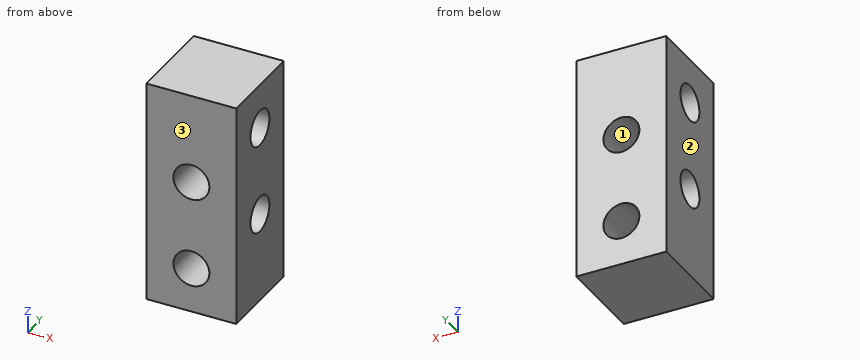
from build123d import *

# Parameters (mm, degrees)
SKETCH_1_W          = 10
SKETCH_1_H          = 10
EXTRUDE_1_DEPTH     = 12.5
SKETCH_2_R          = 2
CUT_EXTRUDE_1_DEPTH = 25
SKETCH_3_R          = 2
CUT_EXTRUDE_2_DEPTH = 25


with BuildPart() as part:
    # 草图1 → 凸台-拉伸1 (new body, symmetric)
    with BuildSketch(Plane.XY):
        Rectangle(SKETCH_1_W, SKETCH_1_H)
    extrude(amount=EXTRUDE_1_DEPTH, both=True)

    # 草图2 → 切除-拉伸1 (cut)
    with BuildSketch(Plane(origin=(5, 0, 0), x_dir=(0, 0, -1), z_dir=(1, 0, 0))):
        with Locations((-7.5, 0)):
            Circle(SKETCH_2_R)
        with Locations((2.5, 0)):
            Circle(SKETCH_2_R)
    extrude(amount=-CUT_EXTRUDE_1_DEPTH, mode=Mode.SUBTRACT)

    # 草图3 → 切除-拉伸2 (cut)
    with BuildSketch(Plane(origin=(0, 5, 0), x_dir=(1, 0, 0), z_dir=(0, 1, 0))):
        with Locations((0, 7.5)):
            Circle(SKETCH_3_R)
        with Locations((0, -2.5)):
            Circle(SKETCH_3_R)
    extrude(amount=-CUT_EXTRUDE_2_DEPTH, mode=Mode.SUBTRACT)


solid = part.part
Geometry: final body of the model. Coordinates: model frame, mm. Face numbers are marked on the shaded views. Give positions to 0.01 mm unless a question says otherwise; leave off trailing zeros. Write each loop counter-clockwise with the first axis right and the second up, starting at its lowest first coordinate (ties: lowest second). Pieces come first, ordered by that corner, then holes.
(1) Mould query, pull axis X, two halves, no side actions, for the marked faces 1, 2 and 3. Classes: released by +X, released by -X, zero draft, split by the parting line, or undercut.
(2) Ray query, line 1 (Z direction, x = 0, y = 2.75); line 2 (X direction, y = -2.75, z = -7.5); line 3 (Z direction, x = 0, y = -0.25). Return the intervals inside material, ascending.
(3) Cut plane B-B, the plane y = 0. Return loops of the section in (x, z).
(4) Cut plane D-D, the plane x = -3.5. Return loops of the section in (y, z), then the cut area to 3 significant figures.
(5) Cut plane A-A, the plane z = 7.5. Return loops of the section in (x, y).
(6) Cut plane C-C, the plane x = 1.25. Return loops of the section in (y, z).
Values follow:
1. face 1: undercut
1. face 2: released by -X
1. face 3: zero draft
2. line 1: z = -12.5 to -9.5, -5.5 to 0.5, 4.5 to 12.5
2. line 2: x = -5 to -2, 2 to 5
2. line 3: z = -12.5 to -9.5, -5.5 to -4.48, -0.52 to 0.5, 4.5 to 5.52, 9.48 to 12.5
3. outline: (-5, -12.5) - (5, -12.5) - (5, -4.5) - (-5, -4.5) - close; (-5, -0.5) - (5, -0.5) - (5, 5.5) - (-5, 5.5) - close; (-5, 9.5) - (5, 9.5) - (5, 12.5) - (-5, 12.5) - close; hole circle Ø4 at (0, -7.5); hole circle Ø4 at (0, 2.5)
4. outline: (-5, -12.5) - (5, -12.5) - (5, 12.5) - (-5, 12.5) - close; hole circle Ø4 at (0, -2.5); hole circle Ø4 at (0, 7.5)
4. area: 225 mm2
5. outline: (-5, -5) - (5, -5) - (5, -2) - (-5, -2) - close; (-5, 2) - (5, 2) - (5, 5) - (-5, 5) - close
6. outline: (-5, -12.5) - (5, -12.5) - (5, -9.06) - (-5, -9.06) - close; (-5, -5.94) - (5, -5.94) - (5, 0.94) - (-5, 0.94) - close; (-5, 4.06) - (5, 4.06) - (5, 12.5) - (-5, 12.5) - close; hole circle Ø4 at (0, -2.5); hole circle Ø4 at (0, 7.5)
